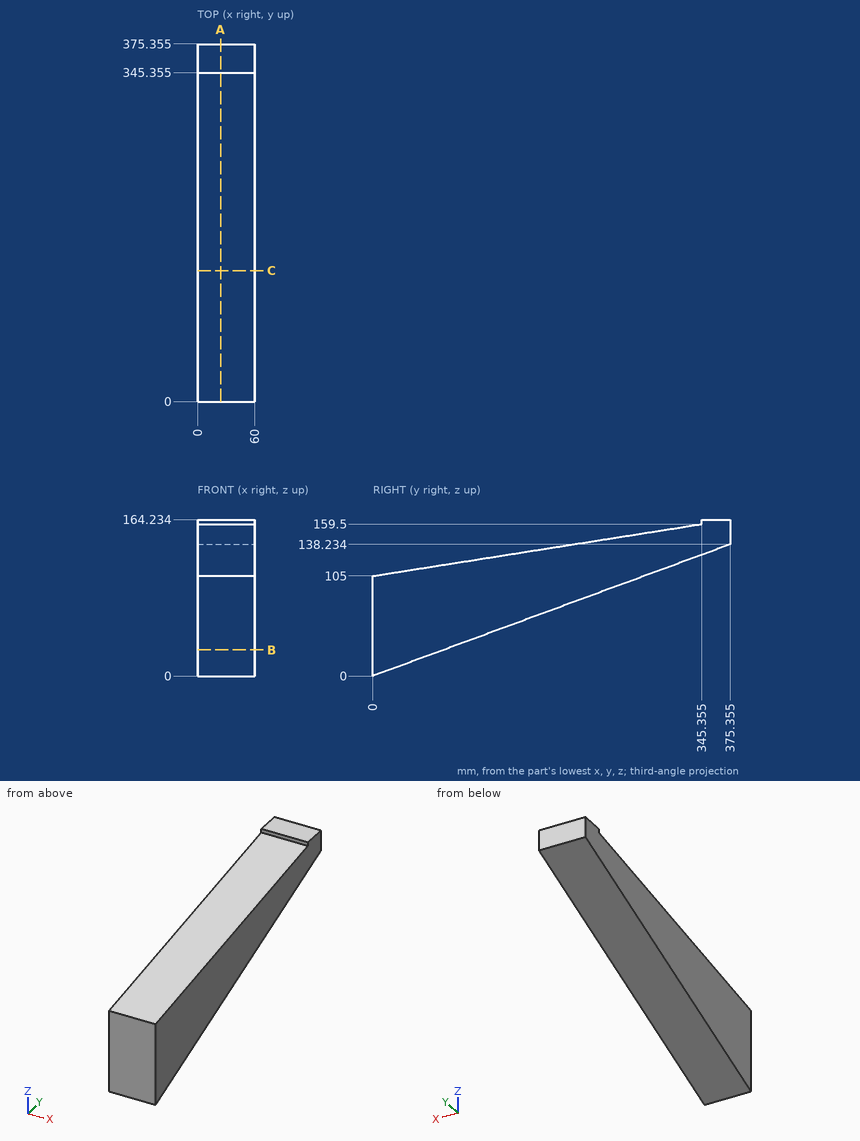
For this review, use the dimensioned drawing (mm, ordinates from the lowest corner) and the shaded views. Give positions to 0.01 mm unless a question says otherwise; leave off trailing zeros. Order: outer loops, then holes, each group sorted by start corner. A loop starts at its lowest first (then second) coordinate and runs counter-clockwise, first axis right, second up. Notation, with made-up numbers: (-7.75, -6.5) - (17.25, -6.5) arc R13 ccw to (17.25, 3.5) - close; hole circle Ø6 at (8.5, -0.5). An arc over 180 degrees is marked (long way). Use CSV: the item, a comma, the result in double quotes. Start each with the question number.
Q1. To check wall thickness, follow line 1 along Z through (x, y) = (54.5, 142) (1 decimal); line 2 along Z through (x, y) = (46.5, 63.5) (1 decimal). State the ranges of each line that lie inside material, in increasing order. Write a range as [from, to].
Q2. Clearance check with flat-ended pins moving along their axes: pin 1 Ø6 at (x, y) = (20.5, 318.5) entering from +Z; pin 2 Ø1.5 at (x, y) = (36, 178.5) entering from +Z; pin 3 Ø1 at (x, y) = (20, 219.5) entering from +Z. State where each tip first meets the part, or that it passes through.
Q3. We need section B-B, the plane z = 27.5. Write out the cut boundary in (x, y), and give its area (3 significant figures).
Q4. We need section A-A, the plane x = 24. Write out the cut boundary in (y, z) (1 decimal), and give its area (3 significant figures).
Q5. We need section C-C, the plane y = 137.5. Write out the cut boundary in (x, z).
Outcome:
1,line 1,"z = [52.3, 127.4]"
1,line 2,"z = [23.4, 115]"
2,pin 1,"stops at z = 155.74"
2,pin 2,"stops at z = 133.29"
2,pin 3,"stops at z = 139.72"
3,outline,"(0, 0) - (60, 0) - (60, 74.67) - (0, 74.67) - close"
3,area,"4,480 mm^2"
4,outline,"(0, 0) - (375.4, 138.2) - (375.4, 164.2) - (345.4, 164.2) - (345.4, 159.5) - (0, 105) - close"
4,area,"24,700 mm^2"
5,outline,"(0, 50.64) - (60, 50.64) - (60, 126.7) - (0, 126.7) - close"
